For this review, use the dimensioned drawing (mm, ordinates from the lowest corner) and the shaded views. A direction names the side the tool comes from. Coordinates: 2 decimals unless noted, no trailing zeros. Loops run counter-clockwise (first coordinate to the right, second up) from the corner with the lowest first, then second, coordinate; pieces in that order, holes last.
1. Take a section at C-C, the plane z = 1.5. State the section outline as (x, y) points.
2. Clearance check with flat-ended pins moving along their axes: P1, Ø1.9, axis at x = 3, z = 7, coming from the -Y side; P2, Ø2, axis at x = 3.95, y = 10.3, coming from the -Z side; P3, Ø1.5, axis at x = 5.5, y = 4, coming from the +Z side. State where each tip first meets the part, or that it passes through.
3. Machinability: for the marked faces 1 and 2, which of the approach directions +Z, -Z, +X, -X, +Y, -Y give a long, thin tool a straight path to every point of the face, cutting with its end or side? Answer none if there is none.
4. Take a section at A-A, the plane y = 10.3. State the section outline as (x, z) points.
5. Take a section at D-D, the plane x = 1.25. State the section outline as (y, z) points, then the cut area to 3 significant figures.
6. Mouldability with a two-part tool opening along X and no side actions: class the marked faces 3, 4, 5 and 6 as pulls with the +X half, pulls with the -X half, needs draft (parallel to the pull), parting line crosses it, or undercut.
7. To check wall thickness, follow probe 1 along X at (y, z) = (10, 4.25); probe 2 along Y at (x, z) = (3.95, 1.9); probe 3 along Y at (x, z) = (4.25, 8.75). State the ranges of each line that lie inside material, in increasing order.
8. Take a section at B-B, the plane x = 3.95. State the section outline as (y, z) points, then the cut area to 4 significant figures.
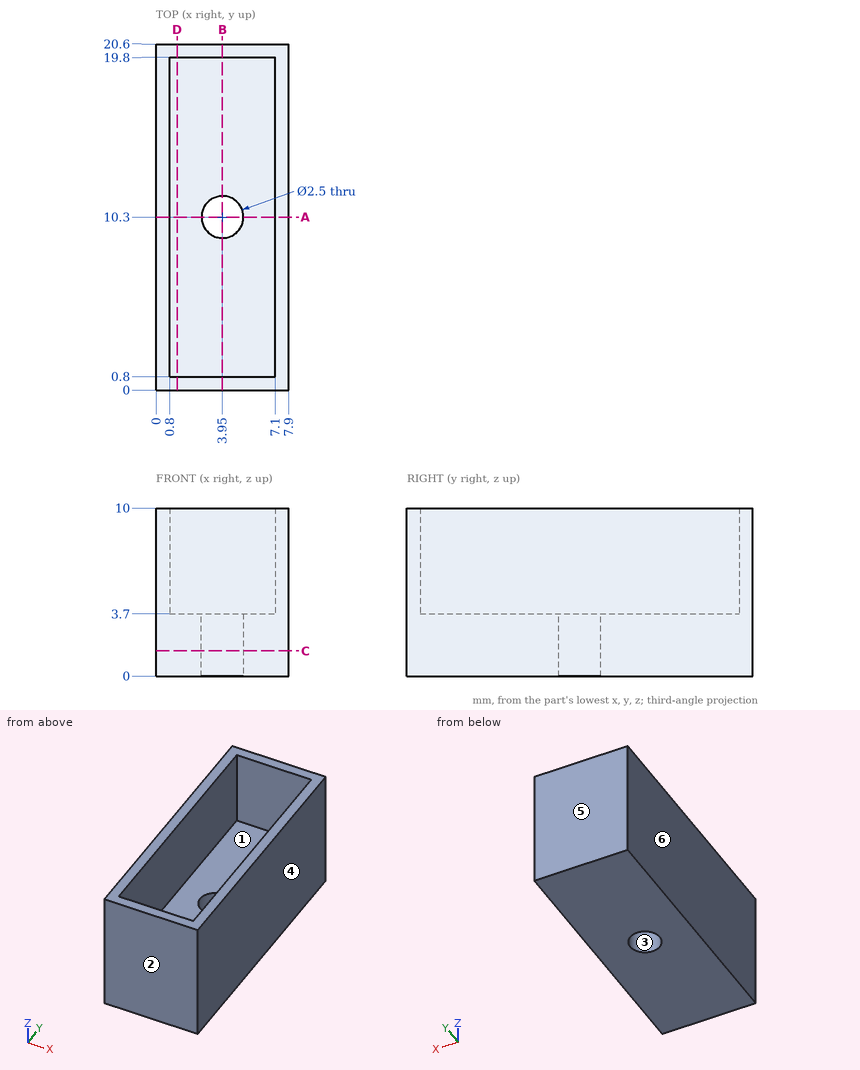
Results list:
1. outline: (0, 0) - (7.9, 0) - (7.9, 20.6) - (0, 20.6) - close; hole circle Ø2.5 at (3.95, 10.3)
2. P1: stops at y = 0
2. P2: passes through
2. P3: stops at z = 3.7
3. face 1: +Z
3. face 2: +Z, -Z, +X, -X, -Y
4. outline: (0, 0) - (2.7, 0) - (2.7, 3.7) - (0.8, 3.7) - (0.8, 10) - (0, 10) - close; (5.2, 0) - (7.9, 0) - (7.9, 10) - (7.1, 10) - (7.1, 3.7) - (5.2, 3.7) - close
5. outline: (0, 0) - (20.6, 0) - (20.6, 10) - (19.8, 10) - (19.8, 3.7) - (0.8, 3.7) - (0.8, 10) - (0, 10) - close
5. area: 86.3 mm2
6. face 3: undercut
6. face 4: pulls with the +X half
6. face 5: needs draft
6. face 6: pulls with the -X half
7. probe 1: x = 0 to 0.8, 7.1 to 7.9
7. probe 2: y = 0 to 9.05, 11.55 to 20.6
7. probe 3: y = 0 to 0.8, 19.8 to 20.6
8. outline: (0, 0) - (9.05, 0) - (9.05, 3.7) - (0.8, 3.7) - (0.8, 10) - (0, 10) - close; (11.55, 0) - (20.6, 0) - (20.6, 10) - (19.8, 10) - (19.8, 3.7) - (11.55, 3.7) - close
8. area: 77.05 mm2
